Could you check a few things on this model? Use its own coordinates, in mm. Coordinates: 2 decimals unless noted, no trailing zeros. Write each loop counter-clockwise with the first axis right and the second up, starting at its lowest first coordinate (ties: lowest second). Pieces come first, ordered by that corner, then holes. Notation, with made-up numbers: M 70.5,2.25 L 93.5,2.25 A9 cw 93.5,10.25 Z; hole C 44,59 d3. An arc over 180 degrees is marked long. Answer as CSV lines item,"result". Start each with the question number.
Item 1: Suppose I cut it at D-D, the plane x = 13.45. State how many separate pieces and enclosed holes the cut face has, and give its area (3 significant figures).
Item 2: I'm going to push flat-ended pins straight in: P1, Ø1.7, axis at x = 2.75, y = 52.64, coming from the -Z side; P2, Ø0.6, axis at y = 89.5, z = 1, coming from the -X side; P3, Ø0.6, axis at x = 2.5, z = 1.5, coming from the -Y side; P4, Ø1, axis at y = 90.5, z = 1, coming from the +X side. Where does each tip first touch, or does it pass through?
Item 3: If I drill on line 1 along X through (y, z) = (52.5, 1.75); line 2 along X through (y, z) = (83.5, 1.1); line 3 along Y through (x, z) = (10, 0.45) (3 decimals), over which ranges is the centre line in solid material (lowest first)? Write a range as [from, to].
Item 4: Suppose I cut it at C-C, the plane y = 45.64. Write out the boundary of the cut face in (x, z), and give its area (3 significant figures).
Item 5: Suppose I cut it at B-B, the plane x = 8.5. Write out the boundary of the cut face in (y, z) (3 decimals), and give its area (3 significant figures).
Item 6: Suppose I cut it at A-A, the plane y = 90. Write out the boundary of the cut face in (x, z).
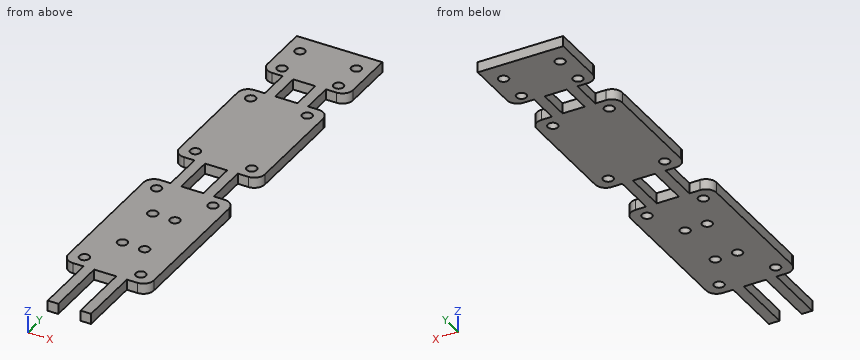
```python
from build123d import *

# Parameters (mm, degrees)
SKETCH1_R           = 0.95
SKETCH1_W           = 4.2
SKETCH1_H           = 8
SKETCH1_H_2         = 6
BOSS_EXTRUDE1_DEPTH = 2


with BuildPart() as part:
    # Sketch1 → Boss-Extrude1 (new body)
    with BuildSketch(Plane.XY):
        with BuildLine():
            Line((4, 26), (2, 26))
            ThreePointArc((2, 26), (0.585786438, 26.585786438), (0, 28))
            Line((0, 28), (0, 53.14))
            ThreePointArc((0, 53.14), (0.585786438, 54.554213562), (2, 55.14))
            Line((2, 55.14), (4, 55.14))
            Line((4, 55.14), (4, 63.14))
            Line((4, 63.14), (2, 63.14))
            ThreePointArc((2, 63.14), (0.585786438, 63.725786438), (0, 65.14))
            Line((0, 65.14), (0, 84.665))
            ThreePointArc((0, 84.665), (0.585786438, 86.079213562), (2, 86.665))
            Line((2, 86.665), (4, 86.665))
            Line((4, 86.665), (4, 92.665))
            Line((4, 92.665), (2, 92.665))
            ThreePointArc((2, 92.665), (0.585786438, 93.250786438), (0, 94.665))
            Line((0, 94.665), (0, 104.46))
            Line((0, 104.46), (16.2, 104.46))
            Line((16.2, 104.46), (16.2, 94.665))
            ThreePointArc((16.2, 94.665), (15.614213562, 93.250786438), (14.2, 92.665))
            Line((14.2, 92.665), (12.2, 92.665))
            Line((12.2, 92.665), (12.2, 86.665))
            Line((12.2, 86.665), (14.2, 86.665))
            ThreePointArc((14.2, 86.665), (15.614213562, 86.079213562), (16.2, 84.665))
            Line((16.2, 84.665), (16.2, 65.14))
            ThreePointArc((16.2, 65.14), (15.614213562, 63.725786438), (14.2, 63.14))
            Line((14.2, 63.14), (12.2, 63.14))
            Line((12.2, 63.14), (12.2, 55.14))
            Line((12.2, 55.14), (14.2, 55.14))
            ThreePointArc((14.2, 55.14), (15.614213562, 54.554213562), (16.2, 53.14))
            Line((16.2, 53.14), (16.2, 28))
            ThreePointArc((16.2, 28), (15.614213562, 26.585786438), (14.2, 26))
            Line((14.2, 26), (12.2, 26))
            Line((12.2, 26), (12.2, 14))
            Line((12.2, 14), (10.2, 14))
            Line((10.2, 14), (10.2, 26))
            Line((10.2, 26), (6, 26))
            Line((6, 26), (6, 14))
            Line((6, 14), (4, 14))
            Line((4, 14), (4, 26))
        make_face()
        with Locations((13.45, 94.665)):
            Circle(SKETCH1_R, mode=Mode.SUBTRACT)
        with Locations((13.45, 84.165)):
            Circle(SKETCH1_R, mode=Mode.SUBTRACT)
        with Locations((13.45, 65.64)):
            Circle(SKETCH1_R, mode=Mode.SUBTRACT)
        with Locations((13.45, 52.64)):
            Circle(SKETCH1_R, mode=Mode.SUBTRACT)
        with Locations((13.45, 28.5)):
            Circle(SKETCH1_R, mode=Mode.SUBTRACT)
        with Locations((10.2, 35.5)):
            Circle(SKETCH1_R, mode=Mode.SUBTRACT)
        with Locations((10.2, 45.64)):
            Circle(SKETCH1_R, mode=Mode.SUBTRACT)
        with Locations((13.45, 100.665)):
            Circle(SKETCH1_R, mode=Mode.SUBTRACT)
        with Locations((2.75, 100.665)):
            Circle(SKETCH1_R, mode=Mode.SUBTRACT)
        with Locations((6, 45.64)):
            Circle(SKETCH1_R, mode=Mode.SUBTRACT)
        with Locations((6, 35.5)):
            Circle(SKETCH1_R, mode=Mode.SUBTRACT)
        with Locations((2.75, 28.5)):
            Circle(SKETCH1_R, mode=Mode.SUBTRACT)
        with Locations((2.75, 52.64)):
            Circle(SKETCH1_R, mode=Mode.SUBTRACT)
        with Locations((2.75, 65.64)):
            Circle(SKETCH1_R, mode=Mode.SUBTRACT)
        with Locations((2.75, 84.165)):
            Circle(SKETCH1_R, mode=Mode.SUBTRACT)
        with Locations((2.75, 94.665)):
            Circle(SKETCH1_R, mode=Mode.SUBTRACT)
        with Locations((8.1, 59.14)):
            Rectangle(SKETCH1_W, SKETCH1_H, mode=Mode.SUBTRACT)
        with Locations((8.1, 89.665)):
            Rectangle(SKETCH1_W, SKETCH1_H_2, mode=Mode.SUBTRACT)
    extrude(amount=BOSS_EXTRUDE1_DEPTH)


solid = part.part
```
Ans:
1,separate pieces,"9"
1,enclosed holes,"0"
1,area,"106 mm^2"
2,P1,"passes through"
2,P2,"stops at x = 4"
2,P3,"stops at y = 26"
2,P4,"stops at x = 12.2"
3,line 1,"x = [0, 1.81], [3.69, 12.51], [14.39, 16.2]"
3,line 2,"x = [0, 2.07], [3.43, 12.77], [14.13, 16.2]"
3,line 3,"y = [26, 34.571], [36.429, 44.711], [46.569, 55.14], [63.14, 86.665], [92.665, 104.46]"
4,outline,"M 0,0 L 5.05,0 L 5.05,2 L 0,2 Z; M 6.95,0 L 9.25,0 L 9.25,2 L 6.95,2 Z; M 11.15,0 L 16.2,0 L 16.2,2 L 11.15,2 Z"
4,area,"24.8 mm^2"
5,outline,"M 26,0 L 55.14,0 L 55.14,2 L 26,2 Z; M 63.14,0 L 86.665,0 L 86.665,2 L 63.14,2 Z; M 92.665,0 L 104.46,0 L 104.46,2 L 92.665,2 Z"
5,area,"129 mm^2"
6,outline,"M 4,0 L 6,0 L 6,2 L 4,2 Z; M 10.2,0 L 12.2,0 L 12.2,2 L 10.2,2 Z"
